```python
from build123d import *

# Parameters (mm, degrees)
F0_R     = 11.049
F0_R_2   = 13.97
F1_DEPTH = 6.35


with BuildPart() as f1:
    # F0 (on Top) → F1 (new body)
    with BuildSketch(Plane.XY):
        with BuildLine():
            ThreePointArc((30.236339, 24.344128), (22.300275, 34.624256), (11.001122, 41.026701))
            ThreePointArc((11.001122, 41.026701), (-9.14954, 42.667843), (-13.198227, 22.86))
            ThreePointArc((-13.198227, 22.86), (-11.642596, 11.421458), (-18.552146, 2.173844))
            ThreePointArc((-18.552146, 2.173844), (-30.464465, 3.49048), (-36.200803, 14.013374))
            ThreePointArc((-36.200803, 14.013374), (-41.135623, 2.000477), (-41.030727, -10.986099))
            ThreePointArc((-41.030727, -10.986099), (-32.376666, -29.257655), (-13.198227, -22.86))
            ThreePointArc((-13.198227, -22.86), (-4.069975, -15.793513), (7.393468, -17.153552))
            ThreePointArc((7.393468, -17.153552), (12.209388, -28.12824), (5.964463, -38.357502))
            ThreePointArc((5.964463, -38.357502), (18.835348, -36.624733), (30.029604, -30.040602))
            ThreePointArc((30.029604, -30.040602), (41.526206, -13.410188), (26.396454, 0))
            ThreePointArc((26.396454, 0), (15.712571, 4.372055), (11.158677, 14.979707))
            ThreePointArc((11.158677, 14.979707), (18.255077, 24.63776), (30.236339, 24.344128))
        make_face()
        with Locations((-26.396454, -15.24)):
            Circle(F0_R, mode=Mode.SUBTRACT)
        Circle(F0_R_2, mode=Mode.SUBTRACT)
        with Locations((26.396454, -15.24)):
            Circle(F0_R, mode=Mode.SUBTRACT)
        with Locations((0, 30.48)):
            Circle(F0_R, mode=Mode.SUBTRACT)
    extrude(amount=F1_DEPTH)


solid = f1.part
```
Could you check a few things on this model? Use its own coordinates, in mm. A direction names the side the tool comes from. Round coordinates to 2 decimals unless told otherwise and drop trailing zeros. Loops run counter-clockwise (first coordinate to the right, second up) from the corner with the lowest first, then second, coordinate; pieces in that order, holes last. Notation, with made-up numbers: (-32.75, -27.5) -> (22.25, -27.5) arc R14 ccw to (22.25, -22.5) -> close; hole circle Ø10 at (-29.75, 61). An arc over 180 degrees is marked (long way). Put each result on its own line as item: value.
Q1. I want a section at C-C on x = -30.5. Write out the boundary of the cut face in (y, z), and give its area (3 significant figures).
Checks:
outline: (-29.92, 0) -> (-25.5, 0) -> (-25.5, 6.35) -> (-29.92, 6.35) -> close; (-4.98, 0) -> (3.51, 0) -> (3.51, 6.35) -> (-4.98, 6.35) -> close
area: 82.0 mm2
Q2. For pin 1 Ø2 at (y, z) = (-14.5, 3.5) entering from -X; pin 2 Ø3 at (x, z) = (1, 4) entering from -Y; pin 3 Ø3 at (x, z) = (-29.5, 2) entering from +Y; pin 4 Ø10 at (x, y) = (-12.5, -21) entering from -Z, each with a flat end and sliding along its axis, tell me the tip position at first contact or that it passes through.
Checks:
pin 1: x = -41.64
pin 2: y = -15.45
pin 3: y = 3.87
pin 4: z = 0
Q3. Which directions (+Z, -Z, +X, -X, +Y, -Y) give clear straight access to the entire face, cutting with the end or side of a thin tool? Please do faces 1 (the cylindrical face through (12.22, -27.95, 3.13)), 2 (the flat face through (-13, 7, 6.35)).
Checks:
face 1: +Z, -Z
face 2: +Z, +X, -X, +Y, -Y
Q4. I want a section at B-B on y = 33. Write out the boundary of the cut face in (x, z), and give its area (3 significant figures).
Checks:
outline: (-15.03, 0) -> (-10.76, 0) -> (-10.76, 6.35) -> (-15.03, 6.35) -> close; (10.76, 0) -> (24.04, 0) -> (24.04, 6.35) -> (10.76, 6.35) -> close
area: 111 mm2
Q5. Please list where these lines run through material, in increasing order: line 1 (Y direction, x = 0, z = 4); line 2 (Y direction, x = 30, z = 4); line 3 (X direction, y = -10.5, z = 1.5). Write a range as from..to.
Checks:
line 1: -15.24..-13.97, 13.97..19.43, 41.53..45.72
line 2: -30.07..-25.68, -4.8..-0.43, 24.47..24.81
line 3: -41.13..-36.38, -16.42..-9.21, 9.21..16.42, 36.38..40.88
Q6. Thinking about a two-plate mould opening in X: for faces 3 (the cylindrical face through (-41.1, 2.18, 3.13)), 4 (the cylindrical face through (-1.438, 41.435, 3.131)), 5 (the cylindrical face through (22.44, 34.5, 3.13)), 6 (the flat face through (-13, 7, 0)), which applies, pulls with the +X half, pulls with the -X half, needs draft (parallel to the pull), parting line crosses it, or undercut?
Checks:
face 3: pulls with the -X half
face 4: undercut
face 5: pulls with the +X half
face 6: needs draft
Q7. I want a section at A-A on x = 0. Write out the boundary of the cut face in (y, z), and give its area (3 significant figures).
Checks:
outline: (-15.24, 0) -> (-13.97, 0) -> (-13.97, 6.35) -> (-15.24, 6.35) -> close; (13.97, 0) -> (19.43, 0) -> (19.43, 6.35) -> (13.97, 6.35) -> close; (41.53, 0) -> (45.72, 0) -> (45.72, 6.35) -> (41.53, 6.35) -> close
area: 69.4 mm2
Q8. I want a section at D-D on z = 3. Write out the boundary of the cut face in (x, y), and give its area (3 significant figures).
Checks:
outline: (-41.03, -10.99) arc R15.24 ccw to (-13.2, -22.86) arc R15.24 cw to (7.39, -17.15) arc R12.96 cw to (5.96, -38.36) arc R32.86 ccw to (30.03, -30.04) arc R15.24 ccw to (26.4, 0) arc R15.24 cw to (11.16, 14.98) arc R12.96 cw to (30.24, 24.34) arc R32.86 ccw to (11, 41.03) arc R15.24 ccw to (-13.2, 22.86) arc R15.24 cw to (-18.55, 2.17) arc R12.96 cw to (-36.2, 14.01) arc R32.86 ccw to start; hole circle Ø22.1 at (-26.4, -15.24); hole circle Ø27.94 at (0, 0); hole circle Ø22.1 at (0, 30.48); hole circle Ø22.1 at (26.4, -15.24)
area: 1,820 mm2
